Input: part model. Units: mm. Frame: model coordinates. A direction names the side the tool comes from. Round coordinates to 2 decimals unless told otherwise and drop trailing zeros. Loops run counter-clockwise (first coordinate to the right, second up) from the corner with the lowest first, then second, coordinate; pieces in that order, holes last.
(1) Access query for faces 1 (the face through (-19.374, -25, 1)), 2 (the face through (-11.022, -25, 4)), 3 (the face through (-3, -25, 7.358)). Directions: +Z, -Z, +X, -X, +Y, -Y. A direction counts if a zero-diameter tool reaches every point of the face in a straight line with its end or side. Return the directions, or none.
(2) Cut plane A-A, the plane x = -22. Output: boundary loops of the cut face in (y, z), and give its area (3 significant figures).
(3) Cut plane C-C, the plane z = 1. Output: boundary loops of the cut face in (x, y), and give its area (3 significant figures).
(4) Cut plane B-B, the plane y = -28. Output: boundary loops of the cut face in (x, z).
(5) Line query: line 1 (X direction, y = -7, z = 4); line 2 (Z direction, x = -21, y = -27); line 3 (X direction, y = -12.5, z = 1.25). Output: solid intervals per line, ascending.
(6) Cut plane D-D, the plane x = -18. Output: boundary loops of the cut face in (y, z).
(7) Draft query along X for faces 4 (the face through (-18, -25, 6.428)), 5 (the face through (-11, -25, 0)), 6 (the face through (-31.261, -25, 4)). Return one class per face: released by +X, released by -X, zero draft, split by the parting line, or undercut.
(8) First-contact query: pin 1 Ø2 at (y, z) = (-30.5, 1) entering from +X; pin 2 Ø0.6 at (y, z) = (-29, 0.5) entering from -X; pin 3 Ø1.5 at (x, y) = (-34, -20) entering from -Z. Flat tips, straight axial feed; report the tip coordinate or a pass-through.
from build123d import *

# Parameters (mm, degrees)
F0_W     = 6.443182
F0_H     = 2.982489
F0_W_2   = 5.090909
F0_H_2   = 3.125394
F1_DEPTH = 50
F2_R     = 1


with BuildPart() as f1:
    # F0 (on Front) → F1 (new body)
    with BuildSketch(Plane.XZ):
        Polygon((-11.21591, 0), (-6.443182, 0), (-6.443182, 7.358421), (-6.443182, 10.34091), (-31.261364, 10.34091), (-31.261364, 7.215516), (-31.261364, 0), (-24.261364, 0), (-19.374487, 0), (-19.374487, 1.973586), (-24.624486, 1.973586), (-24.624486, 6.428131), (-11.022214, 6.428131), (-11.022214, 1.973586), (-15.954031, 1.973586), (-15.954031, 0), align=None)
        with Locations((-3.221591, 8.849666)):
            Rectangle(F0_W, F0_H)
        with Locations((-33.806818, 8.778213)):
            Rectangle(F0_W_2, F0_H_2)
    extrude(amount=F1_DEPTH)

    # F2
    f2_edges = [f1.edges().sort_by_distance(p)[0] for p in [
        (-24.624486, -25, 6.428131),
        (-11.022214, -25, 6.428131),
        (-11.022214, -25, 1.973586),
        (-24.624486, -25, 1.973586),
    ]]
    fillet(f2_edges, radius=F2_R)


solid = f1.part
Reported:
1. face 1: -Z, +Y, -Y
1. face 2: +Y, -Y
1. face 3: -Z, +X, +Y, -Y
2. outline: (-50, 0) - (0, 0) - (0, 1.97) - (-50, 1.97) - close; (-50, 6.43) - (0, 6.43) - (0, 10.34) - (-50, 10.34) - close
2. area: 294 mm2
3. outline: (-31.26, -50) - (-19.37, -50) - (-19.37, 0) - (-31.26, 0) - close; (-15.95, -50) - (-6.44, -50) - (-6.44, 0) - (-15.95, 0) - close
3. area: 1,070 mm2
4. outline: (-36.35, 7.22) - (-31.26, 7.22) - (-31.26, 0) - (-19.37, 0) - (-19.37, 1.97) - (-23.62, 1.97) arc R1 cw to (-24.62, 2.97) - (-24.62, 5.43) arc R1 cw to (-23.62, 6.43) - (-12.02, 6.43) arc R1 cw to (-11.02, 5.43) - (-11.02, 2.97) arc R1 cw to (-12.02, 1.97) - (-15.95, 1.97) - (-15.95, 0) - (-6.44, 0) - (-6.44, 7.36) - (0, 7.36) - (0, 10.34) - (-36.35, 10.34) - close
5. line 1: x = -31.26 to -24.62, -11.02 to -6.44
5. line 2: z = 0 to 1.97, 6.43 to 10.34
5. line 3: x = -31.26 to -19.37, -15.95 to -6.44
6. outline: (-50, 6.43) - (0, 6.43) - (0, 10.34) - (-50, 10.34) - close
7. face 4: undercut
7. face 5: zero draft
7. face 6: released by -X
8. pin 1: stops at x = -6.44
8. pin 2: stops at x = -31.26
8. pin 3: stops at z = 7.22
